```python
from build123d import *

# Parameters (mm, degrees)
F0_W     = 36
F0_H     = 14
F1_DEPTH = 12
F2_W     = 30.7
F2_H     = 8.4
F3_DEPTH = 5
F4_R     = 1.4
F5_DEPTH = 7


# Not quite as in the source:
# - a pattern or mirror of a feature is missing from the dataset's text; its kind, count and spacing are read off the source's solid


with BuildPart() as f1:
    # F0 (on Front) → F1 (new body)
    with BuildSketch(Plane.XZ):
        Rectangle(F0_W, F0_H)
    extrude(amount=F1_DEPTH)

    # F2 (on face) → F3 (cut)
    with BuildSketch(Plane.XZ.offset(12)):
        Rectangle(F2_W, F2_H)
    extrude(amount=-F3_DEPTH, mode=Mode.SUBTRACT)

    # F4 (on face) → F5 (cut, through all)
    with BuildSketch(Plane.XZ.offset(7)):
        with Locations((-10, 0)):
            Circle(F4_R)
    f5 = extrude(amount=-F5_DEPTH, mode=Mode.SUBTRACT)

    # F5_copies: F5 across plane
    add(f5.mirror(Plane(origin=(0, 0, 0), x_dir=(0, 0, 1), z_dir=(1, 0, 0))), mode=Mode.SUBTRACT)


solid = f1.part
```
Input: part model. Units: mm. Frame: model coordinates. A direction names the side the tool comes from. Coordinates: 2 decimals unless noted, no trailing zeros. Write each loop counter-clockwise with the first axis right and the second up, starting at its lowest first coordinate (ties: lowest second). Pieces come first, ordered by that corner, then holes. Notation, with made-up numbers: M 70,-21 L 126,-21 A16 cw 126,-11 Z; hole C -31.5,46 d6. An arc over 180 degrees is marked long. Use one line per item in the form item = value.
Q1. Section A-A (x = -10). Return loops of the section in (y, z).
Answer below:
outline = M -12,-7 L 0,-7 L 0,-1.4 L -7,-1.4 L -7,-4.2 L -12,-4.2 Z; M -12,4.2 L -7,4.2 L -7,1.4 L 0,1.4 L 0,7 L -12,7 Z
Q2. Section B-B (z = 0). Return loops of the section in (x, y).
Answer below:
outline = M -18,-12 L -15.35,-12 L -15.35,-7 L -11.4,-7 L -11.4,0 L -18,0 Z; M -8.6,-7 L 8.6,-7 L 8.6,0 L -8.6,0 Z; M 11.4,-7 L 15.35,-7 L 15.35,-12 L 18,-12 L 18,0 L 11.4,0 Z
Q3. Section C-C (x = 8). Return loops of the section in (y, z).
Answer below:
outline = M -12,-7 L 0,-7 L 0,7 L -12,7 L -12,4.2 L -7,4.2 L -7,-4.2 L -12,-4.2 Z
Q4. Section D-D (z = -2). Return loops of the section in (x, y).
Answer below:
outline = M -18,-12 L -15.35,-12 L -15.35,-7 L 15.35,-7 L 15.35,-12 L 18,-12 L 18,0 L -18,0 Z
Q5. Set-up query: faces 1 (the face through (-15.35, -10, 0)), 2 (the face through (18, -6, 0)). Return all of +Z, -Z, +X, -X, +Y, -Y with unobstructed straight access to the full face (end or side cutting, diameter ignored); none if empty.
Answer below:
face_1 = -Y
face_2 = +Z, -Z, +X, +Y, -Y
Q6. First-contact query: pin 1 (2.5 mm diameter, centred on x = -10, z = 0, fed in from +Y); pin 2 (8 mm diameter, centred on x = 11, z = 3.5, fed in from -Y); pin 3 (4 mm diameter, centred on x = 6.5, z = 2, fed in from -Y). Flat tips, straight axial feed; report the tip coordinate or a pass-through.
Answer below:
pin_1 = through
pin_2 = -12
pin_3 = -7
Q7. Material intervals for probe 1 along X at (y, z) = (-7.75, -1); probe 2 along Z at (x, y) = (10, -5); probe 3 along Y at (x, z) = (-14, 0), sorted ascending. Write a range as from..to.
Answer below:
probe_1 = -18..-15.35, 15.35..18
probe_2 = -7..-1.4, 1.4..7
probe_3 = -7..0
